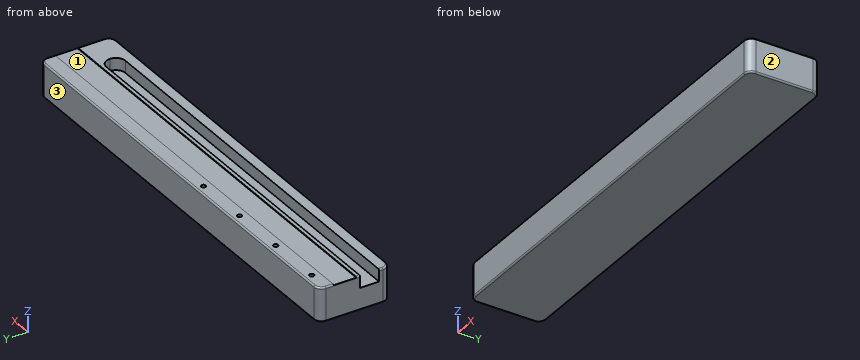
```python
from build123d import *

# Parameters (mm, degrees)
F0_W      = 580
F0_H      = 95
F1_DEPTH  = 45
F3_START  = -40
F2_W      = 25
F2_H      = 16
F3_DEPTH  = 540.001
F6_D      = 6
F6_DEPTH  = 15
F6_TIP    = 1.8025818571
F7_R      = 10
F8_R      = 2
F9_R      = 12.49999
F5_W      = 30
F5_H      = 1
F10_DEPTH = 580.0010001


# Not quite as in the source:
# - a fillet or chamfer is up to 0.001 mm smaller than in the source, because OpenCascade refuses the exact size


with BuildPart() as f1:
    # F0 (on Top) → F1 (new body)
    with BuildSketch(Plane.XY):
        with Locations((43.9460686967, -446.140053056)):
            Rectangle(F0_W, F0_H)
    extrude(amount=F1_DEPTH)

    # F2 (on face) → F3 (cut)
    with BuildSketch(Plane.YZ.offset(333.9460686967).offset(F3_START)):
        with Locations((-466.140053056, 37)):
            Rectangle(F2_W, F2_H)
    extrude(amount=-F3_DEPTH, mode=Mode.SUBTRACT)

    # F6
    with Locations(Plane.XY.offset(45)):
        with Locations((-216.0539313033, -408.640053056), (-141.0539313033, -408.640053056), (-66.0539313033, -408.640053056), (8.9460686967, -408.640053056)):
            Hole(F6_D / 2, depth=F6_DEPTH)
            with Locations((0, 0, -(F6_DEPTH + F6_TIP / 2))):  # 118° drill point
                Cone(0, F6_D / 2, F6_TIP, mode=Mode.SUBTRACT)

    # F7
    f7_edges = [f1.edges().sort_by_distance(p)[0] for p in [
        (-246.053931, -493.640053, 22.5),
        (333.946069, -493.640053, 22.5),
        (333.946069, -398.640053, 22.5),
        (-246.053931, -398.640053, 22.5),
    ]]
    fillet(f7_edges, radius=F7_R)

    # F8
    f8_edges = [f1.edges().sort_by_distance(p)[0] for p in [
        (43.946069, -398.640053, 45),
        (43.946069, -493.640053, 45),
        (43.946069, -493.640053, 0),
    ]]
    fillet(f8_edges, radius=F8_R)

    # F9 (radius 12.5 in the source; OpenCascade refuses exactly that, so slightly less here)
    f9_edges = [f1.edges().sort_by_distance(p)[0] for p in [
        (293.946069, -453.640053, 37),
        (293.946069, -478.640053, 37),
    ]]
    fillet(f9_edges, radius=F9_R)

    # F5 (on face) → F10 (cut, through all)
    with BuildSketch(Plane.YZ.offset(333.9460686967)):
        with Locations((-433.640053056, 44.5)):
            Rectangle(F5_W, F5_H)
    extrude(amount=-F10_DEPTH, mode=Mode.SUBTRACT)


solid = f1.part
```
Verification items for the finished model (mm, model axes). Face numbers are marked on the shaded views. Give positions to 0.01 mm unless a question says otherwise; leave off trailing zeros. Order: outer loops, then holes, each group sorted by start corner. A loop starts at its lowest first (then second) coordinate and runs counter-clockwise, first axis right, second up. Notation, with made-up numbers: (-28.5, 70.25) -> (9.5, 70.25) arc R23 cw to (9.5, 84.25) -> close; hole circle Ø1 at (76, -6). An arc over 180 degrees is marked (long way). Use a Markdown table: item, result.
1) Mould release check, pull along Y, two halves, no side actions. Record for the marked faces 1, 2 and 3: pulls with the +Y half, pulls with the -Y half, needs draft (parallel to the pull), parting line crosses it, or undercut.
Results:
| item | result |
|---|---|
| face 1 | undercut |
| face 2 | needs draft |
| face 3 | pulls with the +Y half |
2) Section check D-D, the plane y = -459.5. Record the boundary of the cut face in (x, z).
Results:
| item | result |
|---|---|
| outline | (-246.05, 2) arc R2 ccw to (-244.05, 0) -> (331.95, 0) arc R2 ccw to (333.95, 2) -> (333.95, 43) arc R2 ccw to (331.95, 45) -> (292.04, 45) -> (292.04, 29) -> (-246.05, 29) -> close |
3) Material ranges on probe 1 along Y at (x, z) = (-46.5, 33); probe 2 along Z at (x, y) = (134.5, -429); probe 3 along Z at (x, y) = (147, -477), recorded low to high.
Results:
| item | result |
|---|---|
| probe 1 | -493.64 to -478.64, -453.64 to -398.64 |
| probe 2 | 0 to 44 |
| probe 3 | 0 to 29 |
4) Depth check by flat-ended pin: pin 1 Ø5 at (x, y) = (-141.05, -408.64) entering from +Z; pin 2 Ø9 at (x, y) = (16.5, -429) entering from +Z; pin 3 Ø1.1 at (x, z) = (159, 44.5) entering from -Y. Enter the tip coordinate at first touch or a pass-through.
Results:
| item | result |
|---|---|
| pin 1 | z = 29.7 |
| pin 2 | z = 44 |
| pin 3 | y = -493.4 |
5) Section check C-C, the plane z = 35. Give the number of separate pieces and of enclosed holes in the cut face, then the cut area to 3 significant figures.
Results:
| item | result |
|---|---|
| separate pieces | 1 |
| enclosed holes | 4 |
| area | 41,500 mm² |
6) Section check A-A, the plane y = -431.5. Record the boundary of the cut face in (x, z).
Results:
| item | result |
|---|---|
| outline | (-246.05, 2) arc R2 ccw to (-244.05, 0) -> (331.95, 0) arc R2 ccw to (333.95, 2) -> (333.95, 43) arc R2 ccw to (333.68, 44) -> (-245.79, 44) arc R2 ccw to (-246.05, 43) -> close |
7) Section check B-B, the plane x = 148. Record the boundary of the cut face in (y, z), then the cut area to 3 significant figures.
Results:
| item | result |
|---|---|
| outline | (-493.64, 2) arc R2 ccw to (-491.64, 0) -> (-400.64, 0) arc R2 ccw to (-398.64, 2) -> (-398.64, 43) arc R2 ccw to (-400.64, 45) -> (-418.64, 45) -> (-418.64, 44) -> (-448.64, 44) -> (-448.64, 45) -> (-453.64, 45) -> (-453.64, 29) -> (-478.64, 29) -> (-478.64, 45) -> (-491.64, 45) arc R2 ccw to (-493.64, 43) -> close |
| area | 3,840 mm² |
